from build123d import *

# Parameters (mm, degrees)
BOSS_EXTRUDE5_DEPTH       = 5
SKETCH9_R                 = 2.2
SKETCH9_R_2               = 1.5
BOSS_EXTRUDE11_DEPTH      = 1.8
BOSS_EXTRUDE11_DEPTH_BACK = 5
SKETCH9_10_R              = 1.5
CUT_EXTRUDE4_DEPTH        = 6
SKETCH11_R                = 2.5
CUT_EXTRUDE5_DEPTH        = 7.8
SKETCH12_W                = 6
SKETCH12_H                = 6
BOSS_EXTRUDE12_DEPTH      = 5
FILLET7_R                 = 0.5


with BuildPart() as part:
    # Sketch8 → Boss-Extrude5 (new body)
    with BuildSketch(Plane.XY):
        with BuildLine():
            Line((-33.540427797, 119.803578872), (10.459572203, 119.803578872))
            ThreePointArc((10.459572203, 119.803578872), (11.873785765, 119.217792435), (12.459572203, 117.803578872))
            Line((12.459572203, 117.803578872), (12.459572203, 87.803578872))
            ThreePointArc((12.459572203, 87.803578872), (11.873785765, 86.38936531), (10.459572203, 85.803578872))
            Line((10.459572203, 85.803578872), (-33.540427797, 85.803578872))
            ThreePointArc((-33.540427797, 85.803578872), (-34.95464136, 86.38936531), (-35.540427797, 87.803578872))
            Line((-35.540427797, 87.803578872), (-35.540427797, 117.803578872))
            ThreePointArc((-35.540427797, 117.803578872), (-34.95464136, 119.217792435), (-33.540427797, 119.803578872))
        make_face()
    extrude(amount=BOSS_EXTRUDE5_DEPTH)

    # Sketch9 → Boss-Extrude11 (add, two sides)
    with BuildSketch(Plane.XY.offset(5)) as boss_extrude11_sk:
        with Locations((-3.540427797, 90.491289859)):
            Circle(SKETCH9_R)
        with Locations((-3.540427797, 90.491289859)):
            Circle(SKETCH9_R_2, mode=Mode.SUBTRACT)
        with Locations((-19.540427797, 90.491289859)):
            Circle(SKETCH9_R)
        with Locations((-19.540427797, 90.491289859)):
            Circle(SKETCH9_R_2, mode=Mode.SUBTRACT)
    extrude(amount=BOSS_EXTRUDE11_DEPTH)
    extrude(boss_extrude11_sk.sketch, amount=-BOSS_EXTRUDE11_DEPTH_BACK)

    # Sketch9<10> → Cut-Extrude4 (cut, through all)
    with BuildSketch(Plane.XY.offset(5)):
        with Locations((-3.540427797, 90.491289859)):
            Circle(SKETCH9_10_R)
        with Locations((-19.540427797, 90.491289859)):
            Circle(SKETCH9_10_R)
    extrude(amount=-CUT_EXTRUDE4_DEPTH, mode=Mode.SUBTRACT)

    # Sketch11 → Cut-Extrude5 (cut, through all)
    with BuildSketch(Plane(origin=(0, 0, 0), x_dir=(-1, 0, 0), z_dir=(0, 0, -1))):
        with Locations((11.540427797, 114.618963942)):
            Circle(SKETCH11_R)
    extrude(amount=-CUT_EXTRUDE5_DEPTH, mode=Mode.SUBTRACT)

    # Sketch12 → Boss-Extrude12 (add)
    with BuildSketch(Plane(origin=(0, 0, 0), x_dir=(-1, 0, 0), z_dir=(0, 0, -1))):
        with Locations((-4.669308543, 98.468963942)):
            Rectangle(SKETCH12_W, SKETCH12_H)
        with Locations((26.892367502, 98.468963942)):
            Rectangle(SKETCH12_W, SKETCH12_H)
    extrude(amount=BOSS_EXTRUDE12_DEPTH)

    # Fillet7
    fillet7_edges = [part.edges().sort_by_distance(p)[0] for p in [
        (-21.740427797, 90.491289859, 6.8),
        (-5.740427797, 90.491289859, 6.8),
    ]]
    fillet(fillet7_edges, radius=FILLET7_R)


solid = part.part
Work out the finished part from the listing and answer in its coordinate system (mm). A direction names the side the tool comes from. Coordinates: 2 decimals unless noted, no trailing zeros. Loops run counter-clockwise (first coordinate to the right, second up) from the corner with the lowest first, then second, coordinate; pieces in that order, holes last. Notation, with made-up numbers: (-35, -31) -> (-1, -31) arc R16 cw to (-1, -4) -> close; hole circle Ø1 at (-21, 48.5). An arc over 180 degrees is marked (long way). Write each question's results on one line, items separated by ' | '. Start each with the question number.
1) Find section A-A on z = -3.5. Determine the outline of the cut face in (x, y), then the cut area to 3 significant figures.
2) Find section C-C on x = 4. Determine the outline of the cut face in (y, z).
3) For faces 1 (the flat face through (-23.892, 98, -2)), 2 (the flat face through (-27, 101.469, -2)), 3 (the cylindrical face through (-20.017, 88.344, 5.641)), determine the directions among +Z, -Z, +X, -X, +Y, -Y from which every point of the face is accessible in a straight line to the end or side of a thin tool.
4) Flat-ended cylindrical pins translate along their axes: P1, Ø5.5, axis at x = -27, z = -2.5, coming from the +Y side; P2, Ø3, axis at x = -11.54, y = 114.62, coming from the +Z side; P3, Ø8, axis at x = -9, y = 115, coming from the +Z side; P4, Ø2.5, axis at y = 99, z = -1.5, coming from the +X side. Find the tip coordinate at first contact, or state that the pin passes through.
5) Find section B-B on y = 100. Determine the outline of the cut face in (x, z).
6) Consider line 1 along Z through (x, y) = (-4.5, 98); line 2 along X through (y, z) = (90, 2.75); line 3 along Y through (x, z) = (2, -0.75). Determine where each line is inside the solid, lowest interval first.
7) The mould has two halves that part along X. Classify faces 4 (the flat face through (1.669, 98, -2)), 5 (the flat face through (5, 101.469, -2)), 6 (the flat face through (-35.54, 103, 2)), 7 (the flat face through (7.669, 98, -2)): pulls with the +X half, pulls with the -X half, needs draft (parallel to the pull), parting line crosses it, or undercut.
8) Find section D-D on z = 4.25. Determine the outline of the cut face in (x, y).
Response values:
1) outline: (-29.89, 95.47) -> (-23.89, 95.47) -> (-23.89, 101.47) -> (-29.89, 101.47) -> close; (1.67, 95.47) -> (7.67, 95.47) -> (7.67, 101.47) -> (1.67, 101.47) -> close | area: 72.0 mm^2
2) outline: (85.8, 0) -> (95.47, 0) -> (95.47, -5) -> (101.47, -5) -> (101.47, 0) -> (119.8, 0) -> (119.8, 5) -> (85.8, 5) -> close
3) face 1: -Z, +Y, -Y | face 2: -Z, +X, -X, +Y | face 3: +Z
4) P1: stops at y = 119.8 | P2: passes through | P3: stops at z = 5 | P4: stops at x = 7.67
5) outline: (-35.54, 0) -> (-29.89, 0) -> (-29.89, -5) -> (-23.89, -5) -> (-23.89, 0) -> (1.67, 0) -> (1.67, -5) -> (7.67, -5) -> (7.67, 0) -> (12.46, 0) -> (12.46, 5) -> (-35.54, 5) -> close
6) line 1: z = 0 to 5 | line 2: x = -35.54 to -20.96, -18.12 to -4.96, -2.12 to 12.46 | line 3: y = 95.47 to 101.47
7) face 4: undercut | face 5: needs draft | face 6: pulls with the -X half | face 7: pulls with the +X half
8) outline: (-35.54, 87.8) arc R2 ccw to (-33.54, 85.8) -> (10.46, 85.8) arc R2 ccw to (12.46, 87.8) -> (12.46, 117.8) arc R2 ccw to (10.46, 119.8) -> (-33.54, 119.8) arc R2 ccw to (-35.54, 117.8) -> close; hole circle Ø3 at (-19.54, 90.49); hole circle Ø5 at (-11.54, 114.62); hole circle Ø3 at (-3.54, 90.49)
